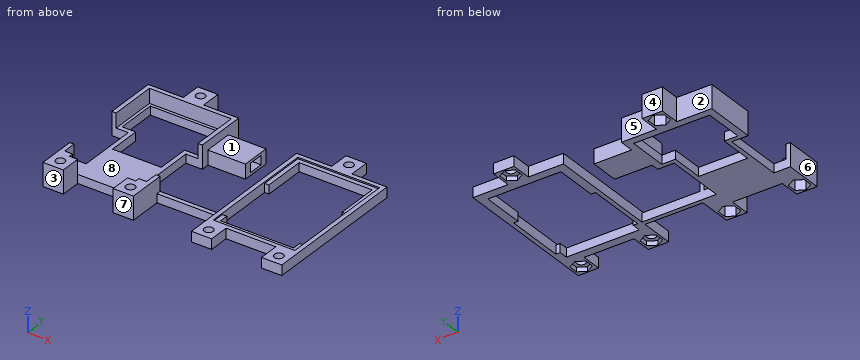
```python
from build123d import *

# Parameters (mm, degrees)
BOSS_EXTRUDE1_DEPTH = 3
BOSS_EXTRUDE2_DEPTH = 5
SKETCH1_4_W         = 13
SKETCH1_4_H         = 10
BOSS_EXTRUDE3_DEPTH = 5
SKETCH2_W           = 3.1
SKETCH2_H           = 5.1
CUT_EXTRUDE1_DEPTH  = 6
SKETCH1_5_W         = 31.2
SKETCH1_5_H         = 44.2
SKETCH1_5_W_2       = 28.248651934
SKETCH1_5_H_2       = 41.207612078
BOSS_EXTRUDE4_DEPTH = 8
SKETCH3_W           = 20
SKETCH3_H           = 1.5
BOSS_EXTRUDE5_DEPTH = 3
SKETCH1_6_W         = 1.475674033
SKETCH1_6_H         = 20.5
CUT_EXTRUDE2_DEPTH  = 25
SKETCH1_7_W         = 1.475674033
SKETCH1_7_H         = 20.5
CUT_EXTRUDE3_DEPTH  = 43.658762289
CUT_EXTRUDE4_DEPTH  = 43.199170608
SKETCH6_W           = 22.86
SKETCH6_H           = 1.496193961
CUT_EXTRUDE5_DEPTH  = 5
BOSS_EXTRUDE6_DEPTH = 3
SKETCH7_4_W         = 7
SKETCH7_4_H         = 7
SKETCH7_4_W_2       = 3.5
BOSS_EXTRUDE8_DEPTH = 3.5
SKETCH8_W           = 7
SKETCH8_H           = 7
BOSS_EXTRUDE9_DEPTH = 8
SKETCH9_R           = 1.55
CUT_EXTRUDE6_DEPTH  = 74.301091397
SKETCH9_3_R         = 1.55
CUT_EXTRUDE7_DEPTH  = 4
SKETCH9_4_R         = 1.55
CUT_EXTRUDE8_DEPTH  = 1.5


with BuildPart() as part:
    # Sketch1 → Boss-Extrude1 (new body)
    with BuildSketch(Plane.XY):
        Polygon((9.93, 4.4), (14.124325967, 4.4), (14.124325967, 20.603806039), (-14.124325967, 20.603806039), (-14.124325967, 4.4), (-9.93, 4.4), (-9.93, -16.1), (-14.124325967, -16.1), (-14.124325967, -20.603806039), (14.124325967, -20.603806039), (14.124325967, -16.1), (9.93, -16.1), align=None)
    extrude(amount=BOSS_EXTRUDE1_DEPTH)

    # Sketch1<3> → Boss-Extrude2 (add)
    with BuildSketch(Plane.XY):
        Polygon((15.6, 22.1), (-15.6, 22.1), (-15.6, -22.1), (15.6, -22.1), (15.6, -16.1), (14.124325967, -16.1), (14.124325967, -20.603806039), (-14.124325967, -20.603806039), (-14.124325967, 20.603806039), (14.124325967, 20.603806039), (14.124325967, 4.4), (15.6, 4.4), align=None)
    extrude(amount=BOSS_EXTRUDE2_DEPTH)

    # Sketch1<4> → Boss-Extrude3 (add)
    with BuildSketch(Plane.XY):
        with Locations((22.1, 12.1)):
            Rectangle(SKETCH1_4_W, SKETCH1_4_H)
    extrude(amount=BOSS_EXTRUDE3_DEPTH)

    # Sketch2 → Cut-Extrude1 (cut)
    with BuildSketch(Plane(origin=(28.6, 0, 0), x_dir=(0, 0, -1), z_dir=(1, 0, 0))):
        with Locations((-2.5, 12.1)):
            Rectangle(SKETCH2_W, SKETCH2_H)
    extrude(amount=-CUT_EXTRUDE1_DEPTH, mode=Mode.SUBTRACT)

    # Sketch1<5> → Boss-Extrude4 (add)
    with BuildSketch(Plane.XY):
        Rectangle(SKETCH1_5_W, SKETCH1_5_H)
        Rectangle(SKETCH1_5_W_2, SKETCH1_5_H_2, mode=Mode.SUBTRACT)
    extrude(amount=BOSS_EXTRUDE4_DEPTH)

    # Sketch3 → Boss-Extrude5 (add)
    with BuildSketch(Plane(origin=(0, 0, 0), x_dir=(-1, 0, 0), z_dir=(0, 0, -1))):
        with Locations((-25.6, -16.85)):
            Rectangle(SKETCH3_W, SKETCH3_H)
    extrude(amount=-BOSS_EXTRUDE5_DEPTH)

    # Sketch1<6> → Cut-Extrude2 (cut)
    with BuildSketch(Plane.XY):
        with Locations((-14.862162984, -5.85)):
            Rectangle(SKETCH1_6_W, SKETCH1_6_H)
    extrude(amount=CUT_EXTRUDE2_DEPTH, mode=Mode.SUBTRACT)

    # Sketch1<7> → Cut-Extrude3 (cut, through all)
    with BuildSketch(Plane.XY):
        with Locations((14.862162984, -5.85)):
            Rectangle(SKETCH1_7_W, SKETCH1_7_H)
    extrude(amount=CUT_EXTRUDE3_DEPTH, mode=Mode.SUBTRACT)

    # Sketch4 → Cut-Extrude4 (cut, through all)
    with BuildSketch(Plane.XY.offset(3)):
        Polygon((-13.124325967, 19.603806039), (13.124325967, 19.603806039), (13.124325967, 5.9), (8.43, 5.9), (8.43, -5.396193961), (-8.43, -5.396193961), (-8.43, 5.9), (-13.124325967, 5.9), align=None)
    extrude(amount=-CUT_EXTRUDE4_DEPTH, mode=Mode.SUBTRACT)

    # Sketch6 → Cut-Extrude5 (cut)
    with BuildSketch(Plane.XY.offset(8)):
        with Locations((0, -21.351903019)):
            Rectangle(SKETCH6_W, SKETCH6_H)
    extrude(amount=-CUT_EXTRUDE5_DEPTH, mode=Mode.SUBTRACT)



with BuildPart() as body_2:
    # Sketch7 → Boss-Extrude6 (new body)
    with BuildSketch(Plane.XY):
        Polygon((51.2, 19.1), (51.2, 20.6), (37.1, 20.6), (37.1, 4.4), (38.6, 4.4), (38.6, 19.1), align=None)
        Polygon((65.3, 20.6), (51.2, 20.6), (51.2, 19.1), (63.8, 19.1), (63.8, 4.4), (65.3, 4.4), align=None)
        Polygon((63.8, -19.1), (51.2, -19.1), (51.2, -20.6), (65.3, -20.6), (65.3, -16.1), (63.8, -16.1), align=None)
        Polygon((51.2, -20.6), (51.2, -19.1), (38.6, -19.1), (38.6, -16.1), (37.1, -16.1), (37.1, -20.6), align=None)
    extrude(amount=BOSS_EXTRUDE6_DEPTH)


with BuildPart() as part_1:
    add(part.part)

    add(body_2.part)  # Boss-Extrude8 merges body 2
    # Sketch7<4> → Boss-Extrude8 (add)
    with BuildSketch(Plane.XY):
        Polygon((47.7, 22.1), (35.6, 22.1), (35.6, -22.1), (42.6, -22.1), (49.2, -22.1), (51.2, -22.1), (51.2, -20.6), (37.1, -20.6), (37.1, -16.1), (37.1, 4.4), (37.1, 20.6), (51.2, 20.6), (51.2, 22.1), align=None)
        Polygon((54.7, 22.1), (51.2, 22.1), (51.2, 20.6), (65.3, 20.6), (65.3, 4.4), (65.3, -16.1), (65.3, -20.6), (51.2, -20.6), (51.2, -22.1), (53.2, -22.1), (59.8, -22.1), (66.8, -22.1), (66.8, 22.1), align=None)
        with Locations((63.3, -25.6)):
            Rectangle(SKETCH7_4_W, SKETCH7_4_H)
        with Locations((39.1, -25.6)):
            Rectangle(SKETCH7_4_W, SKETCH7_4_H)
        with Locations((52.95, 25.6)):
            Rectangle(SKETCH7_4_W_2, SKETCH7_4_H)
        with Locations((49.45, 25.6)):
            Rectangle(SKETCH7_4_W_2, SKETCH7_4_H)
    extrude(amount=BOSS_EXTRUDE8_DEPTH)

    # Sketch8 → Boss-Extrude9 (add)
    with BuildSketch(Plane.XY):
        with Locations((12.1, -25.6)):
            Rectangle(SKETCH8_W, SKETCH8_H)
        with Locations((0, 25.6)):
            Rectangle(SKETCH8_W, SKETCH8_H)
        with Locations((-12.1, -25.6)):
            Rectangle(SKETCH8_W, SKETCH8_H)
    extrude(amount=BOSS_EXTRUDE9_DEPTH)

    # Sketch9 → Cut-Extrude6 (cut, through all)
    with BuildSketch(Plane(origin=(0, 0, 0), x_dir=(-1, 0, 0), z_dir=(0, 0, -1))):
        with Locations((-63.3, -25.6)):
            Circle(SKETCH9_R)
        with Locations((-39.1, -25.6)):
            Circle(SKETCH9_R)
        with Locations((-12.1, -25.6)):
            Circle(SKETCH9_R)
        with Locations((12.1, -25.6)):
            Circle(SKETCH9_R)
        with Locations((0, 25.6)):
            Circle(SKETCH9_R)
        with Locations((-51.2, 25.6)):
            Circle(SKETCH9_R)
    extrude(amount=-CUT_EXTRUDE6_DEPTH, mode=Mode.SUBTRACT)

    # Sketch9<3> → Cut-Extrude7 (cut)
    # profile 1 of 3: a face of its own
    with BuildSketch(Plane(origin=(0, 0, 0), x_dir=(-1, 0, 0), z_dir=(0, 0, -1))):
        Polygon((0, 22.425), (2.749630657, 24.0125), (2.749630657, 27.1875), (0, 28.775), (-2.749630657, 27.1875), (-2.749630657, 24.0125), align=None)
        with Locations((0, 25.6)):
            Circle(SKETCH9_3_R, mode=Mode.SUBTRACT)
    # profile 2 of 3: a face of its own
    with BuildSketch(Plane(origin=(0, 0, 0), x_dir=(-1, 0, 0), z_dir=(0, 0, -1))):
        Polygon((9.350369343, -27.1875), (9.350369343, -24.0125), (12.1, -22.425), (14.849630657, -24.0125), (14.849630657, -27.1875), (12.1, -28.775), align=None)
        with Locations((12.1, -25.6)):
            Circle(SKETCH9_3_R, mode=Mode.SUBTRACT)
    # profile 3 of 3: a face of its own
    with BuildSketch(Plane(origin=(0, 0, 0), x_dir=(-1, 0, 0), z_dir=(0, 0, -1))):
        Polygon((-14.849630657, -27.1875), (-12.1, -28.775), (-9.350369343, -27.1875), (-9.350369343, -24.0125), (-12.1, -22.425), (-14.849630657, -24.0125), align=None)
        with Locations((-12.1, -25.6)):
            Circle(SKETCH9_3_R, mode=Mode.SUBTRACT)
    extrude(amount=-CUT_EXTRUDE7_DEPTH, mode=Mode.SUBTRACT)

    # Sketch9<4> → Cut-Extrude8 (cut)
    # profile 1 of 3: a face of its own
    with BuildSketch(Plane(origin=(0, 0, 0), x_dir=(-1, 0, 0), z_dir=(0, 0, -1))):
        Polygon((-53.949630657, 24.0125), (-51.2, 22.425), (-48.450369343, 24.0125), (-48.450369343, 27.1875), (-51.2, 28.775), (-53.949630657, 27.1875), align=None)
        with Locations((-51.2, 25.6)):
            Circle(SKETCH9_4_R, mode=Mode.SUBTRACT)
    # profile 2 of 3: a face of its own
    with BuildSketch(Plane(origin=(0, 0, 0), x_dir=(-1, 0, 0), z_dir=(0, 0, -1))):
        Polygon((-66.049630657, -27.1875), (-63.3, -28.775), (-60.550369343, -27.1875), (-60.550369343, -24.0125), (-63.3, -22.425), (-66.049630657, -24.0125), align=None)
        with Locations((-63.3, -25.6)):
            Circle(SKETCH9_4_R, mode=Mode.SUBTRACT)
    # profile 3 of 3: a face of its own
    with BuildSketch(Plane(origin=(0, 0, 0), x_dir=(-1, 0, 0), z_dir=(0, 0, -1))):
        Polygon((-41.849630657, -27.1875), (-41.849630657, -24.0125), (-39.1, -22.425), (-36.350369343, -24.0125), (-36.350369343, -27.1875), (-39.1, -28.775), align=None)
        with Locations((-39.1, -25.6)):
            Circle(SKETCH9_4_R, mode=Mode.SUBTRACT)
    extrude(amount=-CUT_EXTRUDE8_DEPTH, mode=Mode.SUBTRACT)


solid = part_1.part
```
Input: part model. Units: mm. Frame: model coordinates. Face numbers are marked on the shaded views. A direction names the side the tool comes from. Coordinates: 2 decimals unless noted, no trailing zeros. Loops run counter-clockwise (first coordinate to the right, second up) from the corner with the lowest first, then second, coordinate; pieces in that order, holes last. Notation, with made-up numbers: (-17, -26) -> (22, -26) arc R13 cw to (22, -9) -> close; hole circle Ø2 at (13.25, 68.25). An arc over 180 degrees is marked (long way). Use a Markdown table: item, result.
1) Cut plane C-C (x = 20). Return the cut outline in (y, z).
Results found:
| item | result |
|---|---|
| outline | (-17.6, 0) -> (-16.1, 0) -> (-16.1, 3) -> (-17.6, 3) -> close; (7.1, 0) -> (17.1, 0) -> (17.1, 5) -> (7.1, 5) -> close |
2) Cut plane D-D (x = 31). Return the cut outline in (y, z), then the cut area to 3 significant figures.
Results found:
| item | result |
|---|---|
| outline | (-17.6, 0) -> (-16.1, 0) -> (-16.1, 3) -> (-17.6, 3) -> close |
| area | 4.50 mm2 |
3) Access query for the marked faces 1, 2, 3, 4 and 5. Directions: +Z, -Z, +X, -X, +Y, -Y. A direction counts if a zero-diameter tool reaches every point of the face in a straight line with its end or side. Return the directions, or none.
Results found:
| item | result |
|---|---|
| face 1 | +Z, +X, +Y, -Y |
| face 2 | +Z, -Z, -X, +Y |
| face 3 | +Z, -Z, +X, -X, -Y |
| face 4 | +Z, -Z, +X, -X, +Y |
| face 5 | +Z, -Z, +Y |
4) Pull-direction query (X, two-part tool) for the marked faces 6, 7 and 8; classes: released by +X, released by -X, zero draft, split by the parting line, or undercut.
Results found:
| item | result |
|---|---|
| face 6 | released by -X |
| face 7 | zero draft |
| face 8 | undercut |
5) Cut plane B-B (y = -8.5). Return the cut outline in (x, z), then the cut area to 3 significant figures.
Results found:
| item | result |
|---|---|
| outline | (-9.93, 0) -> (9.93, 0) -> (9.93, 3) -> (-9.93, 3) -> close; (35.6, 0) -> (37.1, 0) -> (37.1, 3.5) -> (35.6, 3.5) -> close; (65.3, 0) -> (66.8, 0) -> (66.8, 3.5) -> (65.3, 3.5) -> close |
| area | 70.1 mm2 |
6) Contact query for flat-ended pins moving along their axis: pin 1 (1.5 mm diameter, centred on y = 19, z = 5, fed in from +X); pin 2 (4.5 mm diameter, centred on x = 62.5, y = -25, fed in from -Z); pin 3 (3 mm diameter, centred on x = -6.5, z = 4, fed in from +Y); pin 4 (2 mm diameter, centred on x = 26, y = 8.5, fed in from +Z). Output: stop coordinate, or through.
Results found:
| item | result |
|---|---|
| pin 1 | stops at x = 15.6 |
| pin 2 | stops at z = 0 |
| pin 3 | stops at y = 22.1 |
| pin 4 | stops at z = 5 |
7) Cut plane A-A (z = 6.75). Give the number of separate pieces and of enclosed holes in the cut face, then the cut area to 3 significant figures.
Results found:
| item | result |
|---|---|
| separate pieces | 3 |
| enclosed holes | 3 |
| area | 245 mm2 |
8) Material intervals for line 1 along Y through (x, z) = (63.3, 2.25); line 2 along X through (y, z) = (-18.5, 5.5); line 3 along X through (y, z) = (19, 1.25), sorted ascending. Write a range as from..to.
Results found:
| item | result |
|---|---|
| line 1 | y = -29.1..-27.15, -24.05..-19.1, 19.1..22.1 |
| line 2 | x = -15.6..-14.12, 14.12..15.6 |
| line 3 | x = -15.6..-13.12, 13.12..15.6, 35.6..38.6, 63.8..66.8 |
